Work out the finished part from the listing and answer in its coordinate system (mm). Round coordinates to 2 decimals unless told otherwise and drop trailing zeros. Loops run counter-clockwise (first coordinate to the right, second up) from the corner with the lowest first, then second, coordinate; pieces in that order, holes last. Notation, with made-up numbers: (-5.75, 8.5) -> (2.25, 8.5) arc R8 cw to (2.25, 18.5) -> close; hole circle Ø11 at (-36, 38.25). An arc over 180 degrees is marked (long way). Use one line per item in the form item = value.
Autodesk Fusion 360 part; units mm, degrees
sketch "Sketch1" plane through (0, 0, 0) normal (0, 0, 1) x (1, 0, 0)
  circle A0 centre (0, 0) radius 39
  circle A1 centre (0, 0) radius 14
  circle A2 centre (0, 0) radius 17 construction
  circle A3 centre (0, 0) radius 17.5
  circle A4 centre (0, 0) radius 37.5
  line L0 (0, 0) -> (-11.368, 42.4258)
  line L1 (0, 0) -> (43.9224, 0) construction
  line L2 (0, 0) -> (10.4937, -39.163)
  line L3 (0, 0) -> (40.5446, 0) construction
  line L4 (0, 0) -> (-10.0939, -37.6711)
  line L5 (0, 0) -> (39, 0) construction
  line L6 (0, 0) -> (15.1457, 56.5247)
  line L7 (0, 0) -> (58.5186, 0) construction
  line L8 (0, 0) -> (-54.6126, 14.6334)
  line L9 (0, 0) -> (56.5391, 0) construction
  line L10 (0, 0) -> (51.9352, -13.916)
  line L11 (0, 0) -> (53.7673, 0) construction
  line L12 (0, 0) -> (-45.8179, -12.2769)
  line L13 (0, 0) -> (47.4342, 0) construction
  line L14 (0, 0) -> (50.4228, 13.5108)
  line L15 (0, 0) -> (52.2015, 0) construction
  dimension "d1" = 78
  dimension "d2" = 28
  dimension "d3" = 34
  dimension "d32" = 35
  dimension "d33" = 75
  dimension "d34" = 105
  dimension "d35" = 75
  dimension "d36" = 105
  dimension "d37" = 75
  dimension "d38" = 165
  dimension "d39" = 15
  dimension "d40" = 165
  dimension "d41" = 15
extrude "Extrude1" add sketch "Sketch1" along normal blind 4 contours A0 A4 L10 L14 | A0 A4 L6 L14 | A0 A4 L2 L10 | A0 A4 L0 L6 | A3 A4 L6 L14 | A3 A4 L10 L14 | A0 A4 L2 L4 | A3 A4 L2 L10 | A0 A4 L0 L8 | A3 A4 L0 L6 | A1 A3 L6 L14 | A1 A3 L10 L14 | A0 A4 L4 L12 | A3 A4 L2 L4 | A1 A3 L2 L10 | A0 A4 L8 L12 | A3 A4 L0 L8 | A1 A3 L0 L6 | A3 A4 L4 L12 | A1 A3 L2 L4 | A3 A4 L8 L12 | A1 A3 L0 L8 | A1 A3 L4 L12 | A1 A3 L8 L12
sketch "Sketch2" plane through (0, 0, 4) normal (0, 0, 1) x (-1, 0, 0)
  circle A0 centre (0, 0) radius 14
  circle A1 centre (0, 0) radius 39
  line L0 (37, 0) -> (-50, 0) construction
  line L1 (0, -40) -> (0, 43.9283) construction
  circle A2 centre (17, 0) radius 1
  circle A3 centre (0, 17) radius 1
  circle A4 centre (-17, 0) radius 1
  circle A5 centre (0, -17) radius 1
  dimension "d6" = 83.9283
  dimension "d7" = 2
  dimension "d8" = 2
  dimension "d9" = 2
  dimension "d10" = 2
extrude "Extrude2" cut sketch "Sketch2" against normal blind 5 contours A2 | A3 | A4 | A5
sketch "Sketch3" plane through (0, 0, 0) normal (0, 0, 1) x (1, 0, 0)
  circle A0 centre (0, 0) radius 30 construction
  circle A1 centre (30, -0.0028) radius 2.6
  circle A2 centre (0.0015, 30) radius 2.6
  circle A3 centre (-30, -0.0022) radius 2.6
  circle A4 centre (0.0008, -30) radius 2.6
  dimension "d13" = 60
  dimension "d14" = 5.2
  dimension "d15" = 5.2
  dimension "d16" = 5.2
  dimension "d17" = 5.2
extrude "Extrude3" cut sketch "Sketch3" along normal blind 5
sketch "Sketch4" plane through (0, 0, 0) normal (0, 0, 1) x (1, 0, 0)
  circle A0 centre (0, 0) radius 15
  circle A1 centre (0, 0) radius 14
  dimension "d20" = 30
  dimension "d21" = 28
extrude "Extrude4" add sketch "Sketch4" against normal blind 43
extrude "Extrude6" cut sketch "Sketch1" along normal blind 5 contours A3 A4 L6 L14 | A3 A4 L2 L10 | A3 A4 L0 L8 | A3 A4 L4 L12
fillet "Fillet3" radius 2 15 edges at (-9.7057, -36.2222, 2) (9.7057, -36.2222, 2) (-36.2222, -9.7057, 2) (-16.9037, -4.5293, 2) (-4.5293, -16.9037, 2) (-16.9037, 4.5293, 2) (-36.2222, 9.7057, 2) (16.9037, -4.5293, 2) (36.2222, -9.7057, 2) (-9.7057, 36.2222, 2) (-4.5293, 16.9037, 2) (36.2222, 9.7057, 2) (16.9037, 4.5293, 2) (9.7057, 36.2222, 2) (4.5293, 16.9037, 2)
fillet "Fillet4" radius 2 1 edges at (4.5293, -16.9037, 2)
chamfer "Chamfer1" distance 1 angle 45 1 edges at (-13.0526, -5.0626, -43)
chamfer "Chamfer2" distance 1 angle 45 1 edges at (-13.0526, 5.0626, 4)
(1) Find section A-A, the plane x = 0. State how many separate pieces and enclosed holes the cut face has, then the cut area to 3 significant figures.
Completed:
separate_pieces = 6
enclosed_holes = 0
area = 226 mm2
(2) Find section C-C, the plane x = -22. Write down the section's boundary in (y, z), then the cut area to 3 significant figures.
Completed:
outline = (-32.2, 0) -> (-30.37, 0) -> (-30.37, 4) -> (-32.2, 4) -> close; (-5.89, 0) -> (5.89, 0) -> (5.89, 4) -> (-5.89, 4) -> close; (30.37, 0) -> (32.2, 0) -> (32.2, 4) -> (30.37, 4) -> close
area = 61.8 mm2
(3) Find section B-B, the plane y = -31. Write down the section's boundary in (x, z).
Completed:
outline = (-23.66, 0) -> (-21.1, 0) -> (-21.1, 4) -> (-23.66, 4) -> close; (-8.31, 0) -> (-2.4, 0) -> (-2.4, 4) -> (-8.31, 4) -> close; (2.4, 0) -> (8.31, 0) -> (8.31, 4) -> (2.4, 4) -> close; (21.1, 0) -> (23.66, 0) -> (23.66, 4) -> (21.1, 4) -> close
(4) Given P1, Ø1.2, axis at x = 17, y = 0, coming from the -Z side; P2, Ø6, axis at x = 0, y = -30, coming from the -Z side; P3, Ø4, axis at y = -0.5, z = -2.5, coming from the +X side; P4, Ø10, axis at y = 16, z = -20.5, coming from the +X side, each flat-ended and moving along its own axis, determine where each tip first touches the part or whether it passes through.
Completed:
P1 = through
P2 = 0
P3 = 15
P4 = 10.2
(5) Consider L1, parallel to Y at x = 17, z = 3.15; L2, parallel to Y at x = -21.5, z = 1.5. Determine where each line is inside the solid, lowest interval first.
Completed:
L1 = -35.1 to -33.43, -5.37 to -1, 1 to 5.37, 33.43 to 35.1
L2 = -32.54 to -30.72, -5.76 to 5.76, 30.72 to 32.54
(6) Find section D-D, the plane z = -27.5. Write down the section's boundary in (x, y).
Completed:
outline = circle Ø30 at (0, 0); hole circle Ø28 at (0, 0)
